Here's how the part is built. I have some questions about the finished solid (model axes, mm). A direction names the side the tool comes from. Round coordinates to 2 decimals unless told otherwise and drop trailing zeros. Write each loop counter-clockwise with the first axis right and the second up, starting at its lowest first coordinate (ties: lowest second). Pieces come first, ordered by that corner, then holes. Notation, with made-up numbers: (-20.5, -21) -> (20.5, -21) arc R10 cw to (20.5, -17) -> close; hole circle Ø3 at (-13.5, 42). An arc over 180 degrees is marked (long way). Answer as CSV lines item,"result".
from build123d import *

# Parameters (mm, degrees)
F0_R     = 114.3
F1_DEPTH = 165.1
F2_R     = 76.2
F3_DEPTH = 152.4
F4_R     = 10.16
F5_R     = 167.81132
F6_DEPTH = 5.08


with BuildPart() as f1:
    # F0 (on Top) → F1 (new body)
    with BuildSketch(Plane.XY):
        Circle(F0_R)
    extrude(amount=F1_DEPTH)

    # F2 (on face) → F3 (join)
    with BuildSketch(Plane.XY.offset(165.1)):
        Circle(F2_R)
    extrude(amount=F3_DEPTH)

    # F4
    f4_edges = [f1.edges().sort_by_distance(p)[0] for p in [
        (-114.3, 0, 165.1),
        (-76.2, 0, 317.5),
    ]]
    fillet(f4_edges, radius=F4_R)

    # F5 (on face) → F6 (join)
    with BuildSketch(Plane(origin=(0, 0, 0), x_dir=(1, 0, 0), z_dir=(0, 0, -1))):
        Circle(F5_R)
    extrude(amount=F6_DEPTH)


solid = f1.part
Item 1: Suppose I cut it at A-A, the plane x = 0. List the corners of the cut face in (y, z) for me, then the cut area to 3 significant figures.
Results found:
outline,"(-167.81, -5.08) -> (167.81, -5.08) -> (167.81, 0) -> (114.3, 0) -> (114.3, 154.94) arc R10.16 ccw to (104.14, 165.1) -> (76.2, 165.1) -> (76.2, 307.34) arc R10.16 ccw to (66.04, 317.5) -> (-66.04, 317.5) arc R10.16 ccw to (-76.2, 307.34) -> (-76.2, 165.1) -> (-104.14, 165.1) arc R10.16 ccw to (-114.3, 154.94) -> (-114.3, 0) -> (-167.81, 0) -> close"
area,"62,600 mm²"
Item 2: Suppose I cut it at C-C, the plane z = 217. List the corners of the cut face in (x, y) for me, then the cut area to 3 significant figures.
Results found:
outline,"circle Ø152.4 at (0, 0)"
area,"18,200 mm²"
Item 3: Suppose I cut it at D-D, the plane z = 113.5. List the corners of the cut face in (x, y) for me, then the cut area to 3 significant figures.
Results found:
outline,"circle Ø228.6 at (0, 0)"
area,"41,000 mm²"
Item 4: I need wall thicknesses on L1, parallel to Z at x = 12, y = -121.5; L2, parallel to Z at x = -24.5, y = 75; L3, parallel to X at y = 80, z = 57. Which ranges of each line are inside material? Lowest first, please.
Results found:
L1,"z = -5.08 to 0"
L2,"z = -5.08 to 165.1"
L3,"x = -81.64 to 81.64"
Item 5: For faces 1 (the cylindrical face through (-60.47, -46.367, 235.224)), 2 (the cylindrical face through (-21.846, -166.383, -2.504)), which set-ups out of +Z, -Z, +X, -X, +Y, -Y let a thin tool reach every point of the face, with its end or its side?
Results found:
face 1,"+Z"
face 2,"+Z, -Z"
Item 6: Will these pins go through, and if not, where does the flat tip stop? pin 1 (1.5 mm diameter, centred on y = 80, z = 49.5, fed in from +X); pin 2 (2 mm diameter, centred on y = -19, z = 278, fed in from +X); pin 3 (3 mm diameter, centred on x = 31.5, z = 63, fed in from -Y); pin 4 (1.5 mm diameter, centred on x = 116, z = 84.5, fed in from +Y).
Results found:
pin 1,"stops at x = 82.36"
pin 2,"stops at x = 74.04"
pin 3,"stops at y = -110.29"
pin 4,"passes through"
